Here's the drawing with two shaded views (mm, measured from the low corner). I have some questions. A direction names the side the tool comes from. Round coordinates to 2 decimals unless told otherwise and drop trailing zeros. Loops run counter-clockwise (first coordinate to the right, second up) from the corner with the lowest first, then second, coordinate; pieces in that order, holes last. Notation, with made-up numbers: (88.25, -30.5) - (104.25, -30.5) arc R21 cw to (104.25, 4.5) - close; hole circle Ø3 at (-32, 49.5). An arc over 180 degrees is marked (long way). Answer as CSV lines item,"result".
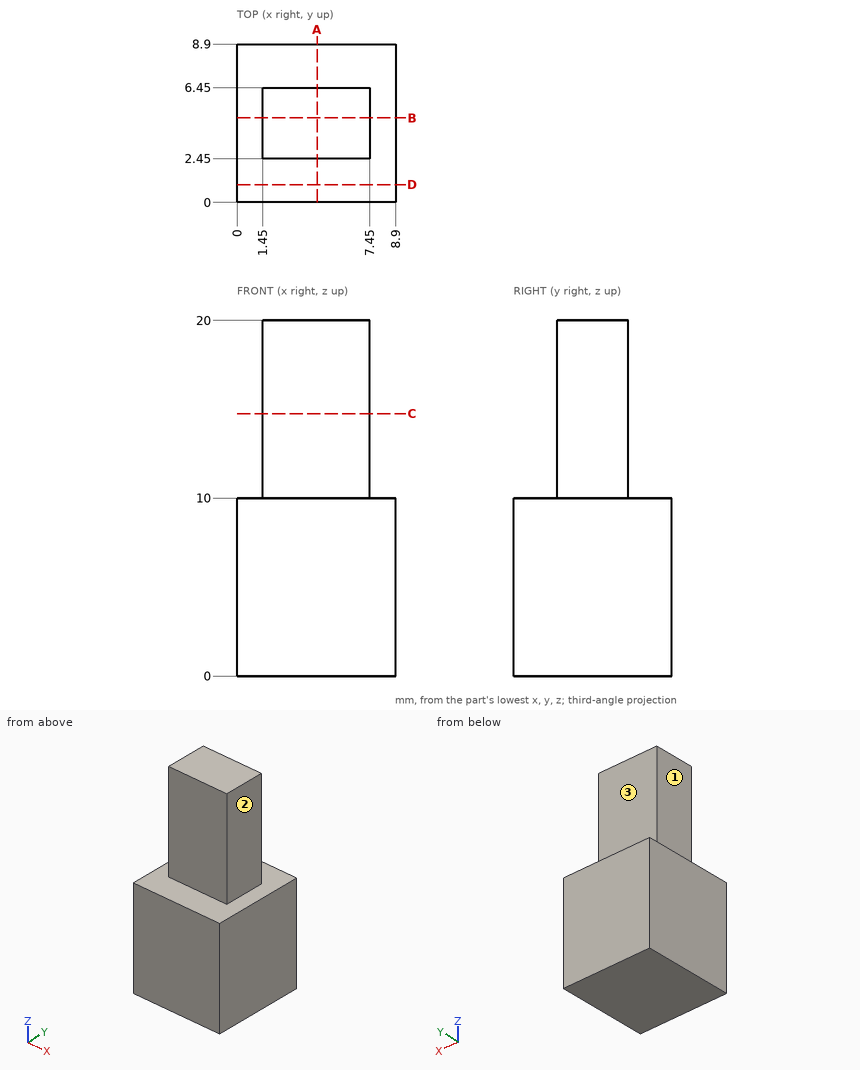
Q1. Imagine slicing it at D-D (y = 1). Write out the boundary of the cut face in (x, z).
Checks:
outline,"(0, 0) - (8.9, 0) - (8.9, 10) - (0, 10) - close"
Q2. Imagine slicing it at A-A (x = 4.5). Write out the boundary of the cut face in (y, z).
Checks:
outline,"(0, 0) - (8.9, 0) - (8.9, 10) - (6.45, 10) - (6.45, 20) - (2.45, 20) - (2.45, 10) - (0, 10) - close"
Q3. Imagine slicing it at C-C (z = 14.75). Write out the boundary of the cut face in (x, y), then the cut area to 3 significant figures.
Checks:
outline,"(1.45, 2.45) - (7.45, 2.45) - (7.45, 6.45) - (1.45, 6.45) - close"
area,"24.0 mm²"
Q4. I'm going to push flat-ended pins straight in: pin 1 Ø3 at (x, z) = (5.5, 13) entering from +Y; pin 2 Ø5 at (y, z) = (4, 11) entering from +X; pin 3 Ø1.2 at (y, z) = (4.5, 17) entering from -X; pin 4 Ø2 at (y, z) = (3.5, 14.5) entering from +X. Where does each tip first touch, or does it pass through?
Checks:
pin 1,"y = 6.45"
pin 2,"x = 8.9"
pin 3,"x = 1.45"
pin 4,"x = 7.45"
Q5. On a 3-axis mill with a long thin cutter (end or side, diameter ignored), from which of +Z, -Z, +X, -X, +Y, -Y can I reach the whole of each face in a straight line? I mean the marked faces 1, 2 and 3. Say none if no direction works.
Checks:
face 1,"+Z, -X, +Y, -Y"
face 2,"+Z, +X, +Y, -Y"
face 3,"+Z, +X, -X, +Y"
Q6. Imagine slicing it at B-B (y = 4.75). Write out the boundary of the cut face in (x, z).
Checks:
outline,"(0, 0) - (8.9, 0) - (8.9, 10) - (7.45, 10) - (7.45, 20) - (1.45, 20) - (1.45, 10) - (0, 10) - close"
Q7. If I drill on line 1 along Y through (x, z) = (2, 13.25); line 2 along Z through (x, y) = (0.75, 2.5); line 3 along X through (y, z) = (5.5, 10.5), over which ranges is the centre line in solid material (lowest first)? Write a range as [from, to].
Checks:
line 1,"[2.45, 6.45]"
line 2,"[0, 10]"
line 3,"[1.45, 7.45]"
